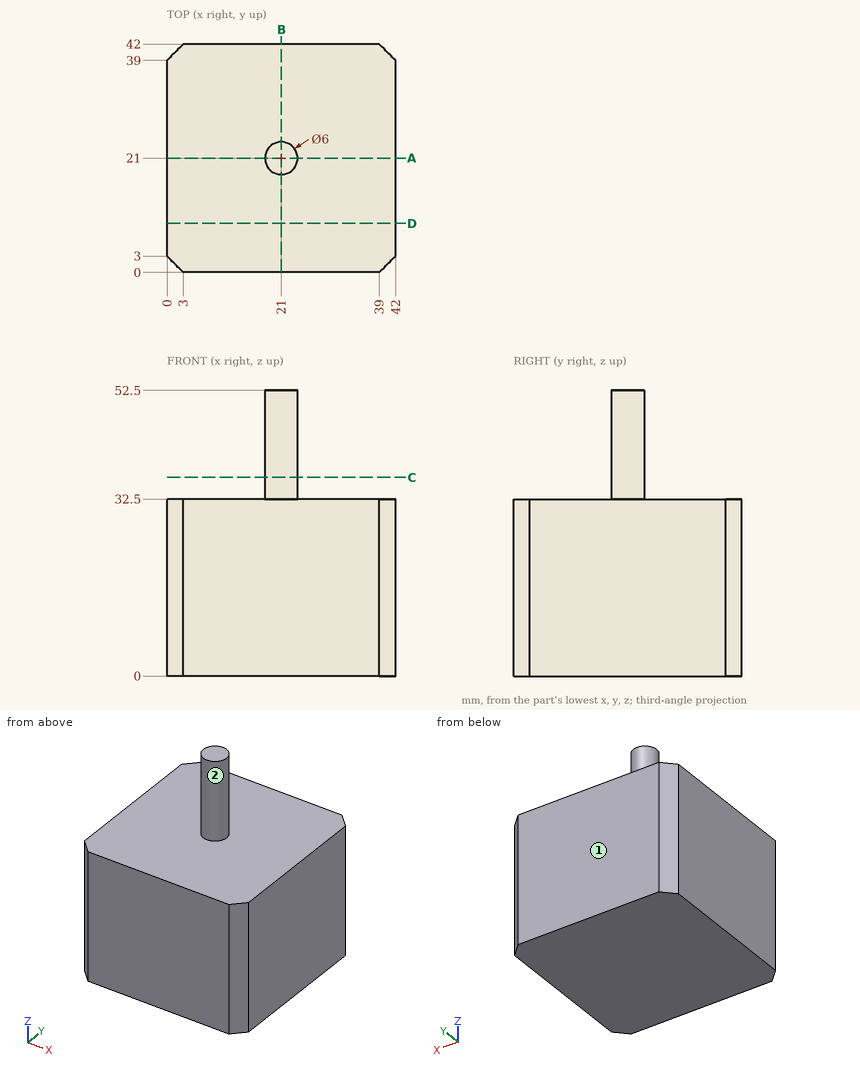
Part print with two shaded views. Sizes in mm from the minimum x, y, z corner. A direction names the side the tool comes from. Coordinates: 2 decimals unless noted, no trailing zeros. Write each loop counter-clockwise with the first axis right and the second up, starting at its lowest first coordinate (ties: lowest second). Pieces come first, ordered by that corner, then holes. Notation, with made-up numbers: (61, 21) - (92, 21) arc R31 cw to (92, 56) - close; hole circle Ø6 at (-33.5, 54). An arc over 180 degrees is marked (long way). Put each result on its own line as item: value.
1. Probe line 1 along Z through (x, y) = (18, 9.5); line 2 along Y through (x, z) = (21, 44); line 3 along X through (y, z) = (40, 23). List the from-to ranges inside material, lowest first. Write a range as [from, to].
Final values:
line 1: z = [0, 32.5]
line 2: y = [18, 24]
line 3: x = [1, 41]
2. Band-saw the part on A-A (y = 21). Write the cut outline in (x, z).
Final values:
outline: (0, 0) - (42, 0) - (42, 32.5) - (24, 32.5) - (24, 52.5) - (18, 52.5) - (18, 32.5) - (0, 32.5) - close
3. Band-saw the part on D-D (y = 9). Write the cut outline in (x, z).
Final values:
outline: (0, 0) - (42, 0) - (42, 32.5) - (0, 32.5) - close
4. Flat gauge pin, fed straight in: pin 1 Ø10 at (x, y) = (16.5, 13.5) entering from +Z. Where does the tip first touch, or does it go through?
Final values:
pin 1: stops at z = 32.5
5. Band-saw the part on C-C (z = 36.5). Write the cut outline in (x, y).
Final values:
outline: circle Ø6 at (21, 21)
6. 3-axis set-ups, long thin cutter, end or side, ignore diameter. For the marked faces 1 and 2: which of +Z, -Z, +X, -X, +Y, -Y reach the whole face in a straight line?
Final values:
face 1: +Z, -Z, +X, -X, +Y
face 2: +Z
